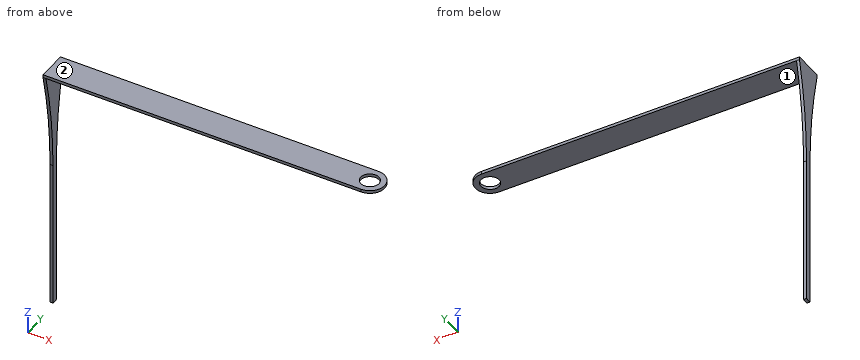
```python
from build123d import *

# Parameters (mm, degrees)
BOSS_EXTRUDE1_DEPTH     = 5
SKETCH2_R               = 5
SKETCH2_R_2             = 3.088913235
BOSS_EXTRUDE2_DEPTH     = 1
SKETCH3_R               = 3.088913235
CUT_EXTRUDE1_DEPTH      = 1
CUT_EXTRUDE2_DEPTH      = 1
CUT_EXTRUDE2_DEPTH_BACK = 10


with BuildPart() as part:
    # Sketch1 → Boss-Extrude1 (new body, symmetric)
    with BuildSketch(Plane(origin=(0, 0, 0), x_dir=(1, 0, 0), z_dir=(0, 1, 0))):
        Polygon((0, 0), (-107, 0), (-107, 84.981911775), (-108, 84.981911775), (-108, -1), (0, -1), align=None)
    extrude(amount=BOSS_EXTRUDE1_DEPTH, both=True)

    # Sketch2 → Boss-Extrude2 (add)
    with BuildSketch(Plane.XY.offset(1)):
        Circle(SKETCH2_R)
        Circle(SKETCH2_R_2, mode=Mode.SUBTRACT)
    extrude(amount=-BOSS_EXTRUDE2_DEPTH)

    # Sketch3 → Cut-Extrude1 (cut)
    with BuildSketch(Plane.XY.offset(1)):
        Circle(SKETCH3_R)
    extrude(amount=-CUT_EXTRUDE1_DEPTH, mode=Mode.SUBTRACT)

    # Sketch4 → Cut-Extrude2 (cut, two sides)
    with BuildSketch(Plane.ZY.offset(108)) as cut_extrude2_sk:
        with BuildLine():
            Line((-84.981911775, 5), (-84.981911775, 1))
            Line((-84.981911775, 1), (-34.527427825, 1))
            ThreePointArc((-34.527427825, 1), (-17.14825011, 2.003332972), (0, 5))
            Line((0, 5), (-84.981911775, 5))
        make_face()
        with BuildLine():
            Line((-34.527427825, -1), (-84.981911775, -1))
            Line((-84.981911775, -1), (-84.981911775, -5))
            Line((-84.981911775, -5), (0, -5))
            ThreePointArc((0, -5), (-17.14825011, -2.003332972), (-34.527427825, -1))
        make_face()
    extrude(amount=CUT_EXTRUDE2_DEPTH, mode=Mode.SUBTRACT)
    extrude(cut_extrude2_sk.sketch, amount=-CUT_EXTRUDE2_DEPTH_BACK, mode=Mode.SUBTRACT)


solid = part.part
```
Here's how the part is built. I have some questions about the finished solid (model axes, mm). Face numbers are marked on the shaded views. A direction names the side the tool comes from. Coordinates: 2 decimals unless noted, no trailing zeros. Order: outer loops, then holes, each group sorted by start corner. A loop starts at its lowest first (then second) coordinate and runs counter-clockwise, first axis right, second up. Notation, with made-up numbers: (37, 11) - (80, 11) arc R20 cw to (80, 37) - close; hole circle Ø11 at (57, -16.75). An arc over 180 degrees is marked (long way). One line per question, with ' | ' between items. Start each with the question number.
1. Please list where these lines run through material, in increasing order: line 1 along X through (y, z) = (0, 0.6); line 2 along Z through (x, y) = (-13, 2); line 3 along X through (y, z) = (0.25, -40.5). Write a range as [from, to].
2. If we section it at A-A (z = -59): Write out the boundary of the cut face in (x, y).
3. If we section it at B-B (x = -79): Write out the boundary of the cut face in (y, z), and give its area (3 significant figures).
4. I'm going to push flat-ended pins straight in: pin 1 Ø3 at (x, y) = (-31.5, 3.5) entering from -Z; pin 2 Ø0.5 at (x, z) = (-107.5, -66.5) entering from +Y; pin 3 Ø0.8 at (x, z) = (-107.5, -50) entering from -Y. Where does each tip first touch, or does it pass through?
5. Which directions (+Z, -Z, +X, -X, +Y, -Y) give clear straight access to the entire face, cutting with the end or side of a thin tool? Please do the marked faces 1 and 2.
Model answer:
1) line 1: x = [-108, -3.09], [3.09, 5] | line 2: z = [0, 1] | line 3: x = [-108, -107]
2) outline: (-108, -1) - (-107, -1) - (-107, 1) - (-108, 1) - close
3) outline: (-5, 0) - (5, 0) - (5, 1) - (-5, 1) - close | area: 10.0 mm²
4) pin 1: stops at z = 0 | pin 2: stops at y = 1 | pin 3: stops at y = -1
5) face 1: -Z, +X, +Y, -Y | face 2: +Z, +X, -X, +Y, -Y
